The listing builds one solid part. Answer for the finished solid, in the listing's coordinates (mm). Coordinates: 2 decimals unless noted, no trailing zeros. Order: outer loops, then holes, each group sorted by start corner. A loop starts at its lowest first (then second) coordinate and runs counter-clockwise, first axis right, second up. Notation, with made-up numbers: (-13, 70) - (44, 70) arc R36 ccw to (44, 105) - close; hole circle Ø4 at (-39.5, 20). An arc over 180 degrees is marked (long way). Use a Markdown table: item, result. Add a question column.
Item 1: The part is cut by section A-A, the plane z = 0. Give the vertices of the cut face in (x, y).
Item 2: The part is cut by section B-B, the plane y = 3.75. Give the vertices of the cut face in (x, z) (3 decimals), then the cut area to 3 significant figures.
Item 3: The part is cut by section D-D, the plane x = -42.5. Give the vertices of the cut face in (y, z).
Item 4: The part is cut by section C-C, the plane z = 33.5. Give the vertices of the cut face in (x, y).
Item 5: Find the intervals of material crossed by line 1 along X through (y, z) = (3.9, 14.5); line 2 along X through (y, z) = (2.65, -1.5); line 3 along Z through (x, y) = (18.5, 1.75), in increasing order.
Item 6: The mould has two halves that part along Z. Classify faces 1 (the flat face through (1, 4.775, -1)), 2 (the cylindrical face through (15.221, 2.354, 48.333)), 3 (the cylindrical face through (-25.947, 2.354, -30.091)), 4 (the cylindrical face through (-34.323, 2.354, 14.425)): released by +Z, released by -Z, zero draft, split by the parting line, or undercut.
Item 7: Flat-ended cylindrical pins translate along their axes: P1, Ø5, axis at x = -37, z = 12.72, coming from the +Y side; P2, Ø1, axis at y = 3.5, z = 23.5, coming from the +X side. Find the tip coordinate at first contact, or state that the pin passes through.
from build123d import *

# Parameters (mm, degrees)
SKETCH1_R           = 50.673
SKETCH1_R_2         = 3.5687
SKETCH1_R_3         = 3.175
BOSS_EXTRUDE1_DEPTH = 4.7752


with BuildPart() as part:
    # Sketch1 → Boss-Extrude1 (new body)
    with BuildSketch(Plane(origin=(0, 0, 0), x_dir=(1, 0, 0), z_dir=(0, 1, 0))):
        with Locations(Location((0, 0, 0), (0, 0, 270))):
            Circle(SKETCH1_R)
        with Locations(Location((-15.875, 0, 0), (0, 0, 270))):
            Circle(SKETCH1_R_2, mode=Mode.SUBTRACT)
        with Locations(Location((15.875, 0, 0), (0, 0, 270))):
            Circle(SKETCH1_R_2, mode=Mode.SUBTRACT)
        with Locations(Location((-37.000474805, -12.718618741, 0), (0, 0, 270))):
            Circle(SKETCH1_R_3, mode=Mode.SUBTRACT)
        with Locations(Location((-23.12973035, 31.556520284, 0), (0, 0, 270))):
            Circle(SKETCH1_R_3, mode=Mode.SUBTRACT)
        with Locations(Location((23.12973035, 31.556520284, 0), (0, 0, 90))):
            Circle(SKETCH1_R_3, mode=Mode.SUBTRACT)
        with Locations(Location((37.000474805, -12.718618741, 0), (0, 0, 90))):
            Circle(SKETCH1_R_3, mode=Mode.SUBTRACT)
    extrude(amount=BOSS_EXTRUDE1_DEPTH)


solid = part.part
Solution:
| question | item | result |
|---|---|---|
| 1 | outline | (-50.67, 0) - (-19.44, 0) - (-19.44, 4.78) - (-50.67, 4.78) - close; (-12.31, 0) - (12.31, 0) - (12.31, 4.78) - (-12.31, 4.78) - close; (19.44, 0) - (50.67, 0) - (50.67, 4.78) - (19.44, 4.78) - close |
| 2 | outline | circle Ø101.346 at (0, 0); hole circle Ø6.35 at (-37, 12.719); hole circle Ø6.35 at (-23.13, -31.557); hole circle Ø7.137 at (-15.875, 0); hole circle Ø7.137 at (15.875, 0); hole circle Ø6.35 at (23.13, -31.557); hole circle Ø6.35 at (37, 12.719) |
| 2 | area | 7,860 mm2 |
| 3 | outline | (0, -27.6) - (4.78, -27.6) - (4.78, 27.6) - (0, 27.6) - close |
| 4 | outline | (-38.02, 0) - (38.02, 0) - (38.02, 4.78) - (-38.02, 4.78) - close |
| 5 | line 1 | x = -48.55 to -39.63, -34.37 to 34.37, 39.63 to 48.55 |
| 5 | line 2 | x = -50.65 to -19.11, -12.64 to 12.64, 19.11 to 50.65 |
| 5 | line 3 | z = -47.18 to -2.42, 2.42 to 47.18 |
| 6 | face 1 | zero draft |
| 6 | face 2 | split by the parting line |
| 6 | face 3 | undercut |
| 6 | face 4 | undercut |
| 7 | P1 | passes through |
| 7 | P2 | stops at x = 45.15 |
